```python
from build123d import *

# Parameters (mm, degrees)
SKETCH_1_R      = 10
SKETCH_1_R_2    = 4
SKETCH_1_R_3    = 1.5
SKETCH_1_R_4    = 2
SKETCH_1_W      = 5.05
SKETCH_1_H      = 2.05
EXTRUDE_1_DEPTH = 2


with BuildPart() as part:
    # 草图1 → 凸台-拉伸1 (new body)
    with BuildSketch(Plane.XY):
        Polygon((317.453360513, 257.462931603), (317.453360513, 258.962931603), (314.853360513, 258.962931603), (314.853360513, 257.462931603), (311.853360513, 257.462931603), (311.853360513, 254.462931603), (314.853360513, 254.462931603), (314.853360513, 252.962931603), (317.453360513, 252.962931603), (317.453360513, 254.462931603), (319.953360513, 254.462931603), (319.953360513, 239.462931603), (321.953360513, 239.462931603), (321.953360513, 234.462931603), (319.953360513, 234.462931603), (319.953360513, 229.462931603), (321.953360513, 229.462931603), (321.953360513, 224.462931603), (319.953360513, 224.462931603), (319.953360513, 219.413055772), (179.953360513, 219.413055772), (179.953360513, 224.462931603), (177.953360513, 224.462931603), (177.953360513, 229.462931603), (179.953360513, 229.462931603), (179.953360513, 234.462931603), (177.953360513, 234.462931603), (177.953360513, 239.462931603), (179.953360513, 239.462931603), (179.953360513, 254.462931603), (182.453360513, 254.462931603), (182.453360513, 252.962931602), (185.053360513, 252.962931602), (185.053360513, 254.462931603), (188.053360513, 254.462931603), (188.053360513, 257.462931603), (185.053360513, 257.462931603), (185.053360513, 258.962931602), (182.453360513, 258.962931602), (182.453360513, 257.462931603), (179.953360513, 257.462931603), (179.953360513, 294.462931603), (182.453360513, 294.462931603), (182.453360513, 292.962931603), (185.053360513, 292.962931603), (185.053360513, 294.462931603), (188.053360513, 294.462931603), (188.053360513, 297.462931603), (185.053360513, 297.462931603), (185.053360513, 298.962931603), (182.453360513, 298.962931603), (182.453360513, 297.462931603), (179.953360513, 297.462931603), (179.953360513, 312.462931603), (177.953360513, 312.462931603), (177.953360513, 317.462931603), (179.953360513, 317.462931603), (179.953360513, 322.462931603), (177.953360513, 322.462931603), (177.953360513, 327.462931603), (179.953360513, 327.462931603), (179.953360513, 338.462931603), (319.953360513, 338.462931603), (319.953360513, 327.462931603), (321.953360513, 327.462931603), (321.953360513, 322.462931603), (319.953360513, 322.462931603), (319.953360513, 317.462931603), (321.953360513, 317.462931603), (321.953360513, 312.462931603), (319.953360513, 312.462931603), (319.953360513, 297.462931603), (317.453360513, 297.462931603), (317.453360513, 298.962931603), (314.853360513, 298.962931603), (314.853360513, 297.462931603), (311.853360513, 297.462931603), (311.853360513, 294.462931603), (314.853360513, 294.462931603), (314.853360513, 292.962931603), (317.453360513, 292.962931603), (317.453360513, 294.462931603), (319.953360513, 294.462931603), (319.953360513, 257.462931603), align=None)
        with Locations((249.953360513, 275.962931603)):
            Circle(SKETCH_1_R, mode=Mode.SUBTRACT)
        with Locations((249.953360513, 255.962931603)):
            Circle(SKETCH_1_R_2, mode=Mode.SUBTRACT)
        with Locations((229.953360513, 335.462931603)):
            Circle(SKETCH_1_R_3, mode=Mode.SUBTRACT)
        with Locations((269.953360513, 335.462931603)):
            Circle(SKETCH_1_R_3, mode=Mode.SUBTRACT)
        with Locations((229.953360513, 255.962931603)):
            Circle(SKETCH_1_R_4, mode=Mode.SUBTRACT)
        with Locations((229.953360513, 295.962931603)):
            Circle(SKETCH_1_R_4, mode=Mode.SUBTRACT)
        with Locations((269.953360513, 295.962931603)):
            Circle(SKETCH_1_R_4, mode=Mode.SUBTRACT)
        with Locations((269.953360513, 255.962931603)):
            Circle(SKETCH_1_R_4, mode=Mode.SUBTRACT)
        with Locations((288.953360513, 335.462931603)):
            Rectangle(SKETCH_1_W, SKETCH_1_H, mode=Mode.SUBTRACT)
        with Locations((298.953360513, 335.462931603)):
            Rectangle(SKETCH_1_W, SKETCH_1_H, mode=Mode.SUBTRACT)
        with Locations((200.953360513, 335.462931603)):
            Rectangle(SKETCH_1_W, SKETCH_1_H, mode=Mode.SUBTRACT)
        with Locations((210.953360513, 335.462931603)):
            Rectangle(SKETCH_1_W, SKETCH_1_H, mode=Mode.SUBTRACT)
    extrude(amount=EXTRUDE_1_DEPTH)


solid = part.part
```
Here's how the part is built. I have some questions about the finished solid (model axes, mm). Give positions to 0.01 mm unless a question says otherwise; leave off trailing zeros. Loops run counter-clockwise (first coordinate to the right, second up) from the corner with the lowest first, then second, coordinate; pieces in that order, holes last. Notation, with made-up numbers: M 44,31.25 L 102,31.25 A31 ccw 102,69.25 Z; hole C 44,-38 d4. An arc over 180 degrees is marked long. Put each result on its own line as item: value. Start each with the question number.
(1) I want a section at A-A on y = 277.5. Please give me the cut outline in (x, z).
(2) I want a section at B-B on z = 0.75. State how many separate pieces and enclosed holes the cut face has, then the cut area to 3 significant figures.
(3) I need wall thicknesses on line 1 along X through (y, z) = (298, 1.35); line 2 along Y through (x, z) = (184, 1.25); line 3 along Y through (x, z) = (210, 0.2). Which ranges of each line are inside material? Lowest first, please. Write a range as [from, to].
(4) If we mould it in two halves opening along X, with no side actions, what happens to faces 1 (the cylindrical face through (231.34, 334.89, 0.99)), 2 (the flat face through (251, 293, 2))? For each: +X half, -X half, draft (parallel to the pull), parting line (faces both ways), or undercut.
(5) Will these pins go through, and if not, where does the flat tip stop? pin 1 Ø1.2 at (y, z) = (254, 1) entering from -X; pin 2 Ø0.6 at (y, z) = (295.5, 1.5) entering from -X; pin 3 Ø0.6 at (x, z) = (320.5, 0.5) entering from -Y.
(6) I want a section at C-C on y = 248. Please give me the cut outline in (x, z).
Answer block:
1. outline: M 179.95,0 L 240.07,0 L 240.07,2 L 179.95,2 Z; M 259.83,0 L 319.95,0 L 319.95,2 L 259.83,2 Z
2. separate pieces: 1
2. enclosed holes: 12
2. area: 16,100 mm^2
3. line 1: [179.95, 182.45], [185.05, 314.85], [317.45, 319.95]
3. line 2: [219.41, 252.96], [258.96, 292.96], [298.96, 338.46]
3. line 3: [219.41, 334.44], [336.49, 338.46]
4. face 1: undercut
4. face 2: draft
5. pin 1: x = 179.95
5. pin 2: x = 188.05
5. pin 3: y = 224.46
6. outline: M 179.95,0 L 319.95,0 L 319.95,2 L 179.95,2 Z
